```python
from build123d import *

# Parameters (mm, degrees)
SKETCH2_W           = 6
SKETCH2_H           = 240
BOSS_EXTRUDE1_DEPTH = 3
BOSS_EXTRUDE2_DEPTH = 240
SKETCH5_W           = 3
SKETCH5_H           = 3
BOSS_EXTRUDE3_DEPTH = 10
SKETCH6_R           = 0.75
CUT_EXTRUDE1_DEPTH  = 40
SKETCH7_W           = 11.65685425
SKETCH7_H           = 10
BOSS_EXTRUDE4_DEPTH = 51.58
SKETCH8_R           = 2.25
BOSS_EXTRUDE5_DEPTH = 12
BOSS_EXTRUDE6_DEPTH = 11.656857
SKETCH10_R          = 3.5
BOSS_EXTRUDE7_DEPTH = 2


with BuildPart() as part:
    # Sketch2 → Boss-Extrude1 (new body)
    with BuildSketch(Plane.XY):
        with Locations((-3, -120)):
            Rectangle(SKETCH2_W, SKETCH2_H)
    extrude(amount=BOSS_EXTRUDE1_DEPTH)

    # Sketch4 → Boss-Extrude2 (add)
    with BuildSketch(Plane(origin=(0, -240, 0), x_dir=(-1, 0, 0), z_dir=(0, -1, 0))):
        Polygon((0, 0), (-2.828427125, 2.828427125), (-2.828427125, -3), (0, -3), align=None)
        Polygon((8.828427125, -3), (6, -3), (6, 0), (8.828427125, 2.828427125), align=None)
    extrude(amount=-BOSS_EXTRUDE2_DEPTH)

    # Sketch5 → Boss-Extrude3 (add)
    with BuildSketch(Plane(origin=(0, 0, 0), x_dir=(1, 0, 0), z_dir=(0, 1, 0))):
        with Locations((-6.5, -1.5)):
            Rectangle(SKETCH5_W, SKETCH5_H)
        with Locations((0.5, -1.5)):
            Rectangle(SKETCH5_W, SKETCH5_H)
    extrude(amount=BOSS_EXTRUDE3_DEPTH)

    # Sketch6 → Cut-Extrude1 (cut)
    with BuildSketch(Plane(origin=(2, 0, 0), x_dir=(0, 0, -1), z_dir=(1, 0, 0))):
        with Locations((-1.5, 6)):
            Circle(SKETCH6_R)
    extrude(amount=-CUT_EXTRUDE1_DEPTH, mode=Mode.SUBTRACT)

    # Sketch7 → Boss-Extrude4 (add)
    with BuildSketch(Plane(origin=(0, 0, 0), x_dir=(-1, 0, 0), z_dir=(0, 0, -1))):
        with Locations((3, -235)):
            Rectangle(SKETCH7_W, SKETCH7_H)
    extrude(amount=BOSS_EXTRUDE4_DEPTH)

    # Sketch8 → Boss-Extrude5 (add)
    with BuildSketch(Plane(origin=(0, 0, -51.58), x_dir=(-1, 0, 0), z_dir=(0, 0, -1))):
        with Locations((3, -235)):
            Circle(SKETCH8_R)
    extrude(amount=BOSS_EXTRUDE5_DEPTH)

    # Sketch9 → Boss-Extrude6 (add)
    with BuildSketch(Plane.ZY.offset(8.828427125)):
        Polygon((-7, -230), (0, -230), (0, -223), align=None)
    extrude(amount=-BOSS_EXTRUDE6_DEPTH)

    # Sketch10 → Boss-Extrude7 (add)
    with BuildSketch(Plane(origin=(0, 0, -51.58), x_dir=(-1, 0, 0), z_dir=(0, 0, -1))):
        with Locations((3, -235)):
            Circle(SKETCH10_R)
    extrude(amount=BOSS_EXTRUDE7_DEPTH)


solid = part.part
```
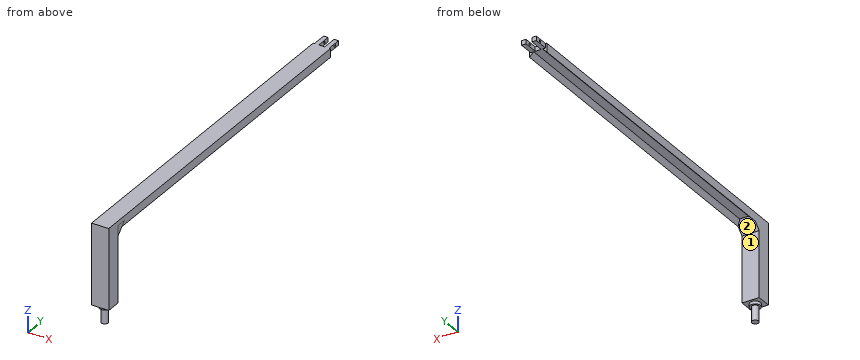
Design review of the part built by this model. Coordinates are the model's own, in mm. Face numbers are marked on the shaded views. Round coordinates to 2 decimals unless told otherwise and drop trailing zeros. Write each loop counter-clockwise with the first axis right and the second up, starting at its lowest first coordinate (ties: lowest second). Pieces come first, ordered by that corner, then holes. Notation, with made-up numbers: (-24, 8.25) -> (25, 8.25) arc R27 ccw to (25, 29.25) -> close; hole circle Ø11 at (-33, -9). An arc over 180 degrees is marked (long way). Answer in a Markdown table with one row per item.
Q1. Take a section at A-A, the plane y = -235. State the section outline as (x, z) points, then the cut area to 3 significant figures.
The answers:
| item | result |
|---|---|
| outline | (-8.83, -51.58) -> (-6.5, -51.58) -> (-6.5, -53.58) -> (-5.25, -53.58) -> (-5.25, -63.58) -> (-0.75, -63.58) -> (-0.75, -53.58) -> (0.5, -53.58) -> (0.5, -51.58) -> (2.83, -51.58) -> (2.83, 3) -> (-8.83, 3) -> close |
| area | 695 mm² |
Q2. To check wall thickness, follow L1, parallel to Y at x = 0.2, z = 1.5; L2, parallel to Y at x = -3.5, z = -48; L3, parallel to Z at x = -5.75, y = -212.5. State the ranges of each line that lie inside material, in increasing order. Write a range as [from, to].
The answers:
| item | result |
|---|---|
| L1 | [-240, 5.25], [6.75, 10] |
| L2 | [-240, -230] |
| L3 | [0, 3] |
Q3. Take a section at B-B, the plane x = -3. State the section outline as (y, z) points, then the cut area to 3 significant figures.
The answers:
| item | result |
|---|---|
| outline | (-240, -51.58) -> (-238.5, -51.58) -> (-238.5, -53.58) -> (-237.25, -53.58) -> (-237.25, -63.58) -> (-232.75, -63.58) -> (-232.75, -53.58) -> (-231.5, -53.58) -> (-231.5, -51.58) -> (-230, -51.58) -> (-230, -7) -> (-223, 0) -> (0, 0) -> (0, 3) -> (-240, 3) -> close |
| area | 1,320 mm² |
Q4. Clearance check with flat-ended pins moving along their axes: pin 1 Ø5 at (x, y) = (-5.5, -103.5) entering from -Z; pin 2 Ø0.9 at (y, z) = (7, 2) entering from -X; pin 3 Ø1.5 at (x, y) = (-4, -91.5) entering from -Z. State where each tip first meets the part, or that it passes through.
The answers:
| item | result |
|---|---|
| pin 1 | z = -2 |
| pin 2 | x = -8 |
| pin 3 | z = 0 |
Q5. Draft analysis for pull direction X (two halves, no side actions). For the marked faces 1 and 2, state which applies: +X half, -X half, draft (parallel to the pull), parting line (faces both ways), or undercut.
The answers:
| item | result |
|---|---|
| face 1 | draft |
| face 2 | undercut |
Q6. Take a section at C-C, the plane z = -57. State the section outline as (x, y) points.
The answers:
| item | result |
|---|---|
| outline | circle Ø4.5 at (-3, -235) |
Q7. Take a section at D-D, the plane y = -55. State the section outline as (x, z) points.
The answers:
| item | result |
|---|---|
| outline | (-8.83, -2.83) -> (-6, 0) -> (0, 0) -> (2.83, -2.83) -> (2.83, 3) -> (-8.83, 3) -> close |
